CAD build for the part. Positions are in the model's coordinates, mm. Face numbers are marked on the shaded views. A direction names the side the tool comes from. Round coordinates to 2 decimals unless told otherwise and drop trailing zeros. Order: outer loops, then holes, each group sorted by start corner. A loop starts at its lowest first (then second) coordinate and runs counter-clockwise, first axis right, second up. Notation, with made-up numbers: (-4, -35) - (2, -35) arc R26 cw to (2, 0) - close; hole circle Ø8 at (54.5, 3.25). An arc over 180 degrees is marked (long way). Write item = value, one per line.
from build123d import *

# Parameters (mm, degrees)
SKETCH1_W                                 = 101.6
SKETCH1_H                                 = 101.6
BASE_EXTRUDE_DEPTH                        = 3.175
SKETCH9_R                                 = 34.925
CENTER_HOLE_DEPTH                         = 29.575
SKETCH2_R                                 = 5.715
SKETCH2_R_2                               = 3.175
LEFT_HINGE_BASE_DEPTH                     = 50.8
LEFT_HINGE_BASE_DEPTH_BACK                = 50.8
SKETCH2_3_R                               = 3.175
LEFT_HINGE_CUT_DEPTH                      = 50.8
LEFT_HINGE_CUT_DEPTH_BACK                 = 50.8
SKETCH3_W                                 = 101.6
SKETCH3_H                                 = 6.35
LEFT_HINGE_EXTENSION_DEPTH                = 3.503095
SKETCH4_R                                 = 5.715
SKETCH4_R_2                               = 3.175
BACK_HINGE_BASE_DEPTH                     = 50.8
BACK_HINGE_BASE_DEPTH_BACK                = 50.8
SKETCH4_3_R                               = 3.175
BACK_HINGE_CUT_DEPTH                      = 50.8
BACK_HINGE_CUT_DEPTH_BACK                 = 50.8
SKETCH7_W                                 = 101.6
SKETCH7_H                                 = 6.35
BACK_HINGE_EXTENSION_DEPTH                = 3.503095
SKETCH8_W                                 = 13.006904881
SKETCH8_H                                 = 12.7
HINGE_CUT_LEFT_DEPTH                      = 32.115
HINGE_CUT_LEFT_LPATTERN_COUNT             = 4
HINGE_CUT_LEFT_LPATTERN_PITCH             = 25.4
HINGE_CUT_BACK_CIRPATTERN_COUNT           = 2
HINGE_CUT_BACK_CIRPATTERN_ANGLE           = 90
HINGE_CUT_BACK_CIRPATTERN_COPY_1_SKETCH_W = 13.006904881
HINGE_CUT_BACK_CIRPATTERN_COPY_1_SKETCH_H = 12.7
HINGE_CUT_BACK_CIRPATTERN_COPY_1_DEPTH    = 32.115
HINGE_CUT_BACK_CIRPATTERN_COPY_2_SKETCH_W = 13.006904881
HINGE_CUT_BACK_CIRPATTERN_COPY_2_SKETCH_H = 12.7
HINGE_CUT_BACK_CIRPATTERN_COPY_2_DEPTH    = 32.115
HINGE_CUT_BACK_CIRPATTERN_COPY_3_SKETCH_W = 13.006904881
HINGE_CUT_BACK_CIRPATTERN_COPY_3_SKETCH_H = 12.7
HINGE_CUT_BACK_CIRPATTERN_COPY_3_DEPTH    = 32.115
CIRPATTERN2_COPY_1_SKETCH_W               = 13.006904881
CIRPATTERN2_COPY_1_SKETCH_H               = 12.7
CIRPATTERN2_COPY_1_DEPTH                  = 32.115
CIRPATTERN2_COPY_2_SKETCH_W               = 13.006904881
CIRPATTERN2_COPY_2_SKETCH_H               = 12.7
CIRPATTERN2_COPY_2_DEPTH                  = 32.115
CIRPATTERN2_COPY_3_SKETCH_W               = 13.006904881
CIRPATTERN2_COPY_3_SKETCH_H               = 12.7
CIRPATTERN2_COPY_3_DEPTH                  = 32.115
CIRPATTERN2_COPY_4_SKETCH_W               = 13.006904881
CIRPATTERN2_COPY_4_SKETCH_H               = 12.7
CIRPATTERN2_COPY_4_DEPTH                  = 32.115


with BuildPart() as part:
    # Sketch1 → Base Extrude (new body, symmetric)
    with BuildSketch(Plane(origin=(0, 0, 0), x_dir=(1, 0, 0), z_dir=(0, 1, 0))):
        Rectangle(SKETCH1_W, SKETCH1_H)
    extrude(amount=BASE_EXTRUDE_DEPTH, both=True)

    # Sketch9 → Center Hole (cut, through all)
    with BuildSketch(Plane(origin=(0, 25.4, 0), x_dir=(-1, 0, 0), z_dir=(0, 1, 0))):
        with Locations(Location((0, 0, 0), (0, 0, 90))):  # turned: the seam where the file's is
            Circle(SKETCH9_R)
    extrude(amount=-CENTER_HOLE_DEPTH, mode=Mode.SUBTRACT)



with BuildPart() as body_2:
    # Sketch2 → Left Hinge Base (new body, two sides)
    with BuildSketch(Plane.XY) as left_hinge_base_sk:
        with Locations((-59.055, 0)):
            Circle(SKETCH2_R)
        with Locations((-59.055, 0)):
            Circle(SKETCH2_R_2, mode=Mode.SUBTRACT)
        with Locations((-59.055, 0)):
            Circle(SKETCH2_R_2)
    extrude(amount=LEFT_HINGE_BASE_DEPTH)
    extrude(left_hinge_base_sk.sketch, amount=-LEFT_HINGE_BASE_DEPTH_BACK)

    # Sketch2_3 → Left Hinge Cut (cut, two sides)
    with BuildSketch(Plane.XY) as left_hinge_cut_sk:
        with Locations((-59.055, 0)):
            Circle(SKETCH2_3_R)
    extrude(amount=LEFT_HINGE_CUT_DEPTH, mode=Mode.SUBTRACT)
    extrude(left_hinge_cut_sk.sketch, amount=-LEFT_HINGE_CUT_DEPTH_BACK, mode=Mode.SUBTRACT)


with BuildPart() as part_1:
    add(part.part)

    add(body_2.part)  # Left Hinge Extension merges body 2
    # Sketch3 → Left Hinge Extension (add)
    with BuildSketch(Plane.ZY.offset(50.8)):
        Rectangle(SKETCH3_W, SKETCH3_H)
    extrude(amount=LEFT_HINGE_EXTENSION_DEPTH)



with BuildPart() as body_2_2:
    # Sketch4 → Back Hinge Base (new body, two sides)
    with BuildSketch(Plane(origin=(0, 0, 0), x_dir=(0, 0, -1), z_dir=(1, 0, 0))) as back_hinge_base_sk:
        with Locations((59.055, 0)):
            Circle(SKETCH4_R)
        with Locations((59.055, 0)):
            Circle(SKETCH4_R_2, mode=Mode.SUBTRACT)
        with Locations((59.055, 0)):
            Circle(SKETCH4_R_2)
    extrude(amount=BACK_HINGE_BASE_DEPTH)
    extrude(back_hinge_base_sk.sketch, amount=-BACK_HINGE_BASE_DEPTH_BACK)

    # Sketch4_3 → Back Hinge Cut (cut, two sides)
    with BuildSketch(Plane(origin=(0, 0, 0), x_dir=(0, 0, -1), z_dir=(1, 0, 0))) as back_hinge_cut_sk:
        with Locations((59.055, 0)):
            Circle(SKETCH4_3_R)
    extrude(amount=BACK_HINGE_CUT_DEPTH, mode=Mode.SUBTRACT)
    extrude(back_hinge_cut_sk.sketch, amount=-BACK_HINGE_CUT_DEPTH_BACK, mode=Mode.SUBTRACT)


with BuildPart() as part_2:
    add(part_1.part)

    add(body_2_2.part)  # Back Hinge Extension merges body 2 2
    # Sketch7 → Back Hinge Extension (add)
    with BuildSketch(Plane(origin=(0, 0, -50.8), x_dir=(-1, 0, 0), z_dir=(0, 0, -1))):
        Rectangle(SKETCH7_W, SKETCH7_H)
    extrude(amount=BACK_HINGE_EXTENSION_DEPTH)

    # Sketch8 → Hinge Cut Left (cut, through all)
    with BuildSketch(Plane(origin=(0, 25.4, 0), x_dir=(-1, 0, 0), z_dir=(0, 1, 0))):
        with Locations((58.26654756, 44.45)):
            Rectangle(SKETCH8_W, SKETCH8_H)
    hinge_cut_left = extrude(amount=-HINGE_CUT_LEFT_DEPTH, mode=Mode.SUBTRACT)

    # Hinge Cut Left LPattern: Hinge Cut Left ×4
    with Locations(*[(0, 0, -i * HINGE_CUT_LEFT_LPATTERN_PITCH) for i in range(1, HINGE_CUT_LEFT_LPATTERN_COUNT)]):
        add(hinge_cut_left, mode=Mode.SUBTRACT)

    # Hinge Cut Back CirPattern: Hinge Cut Left ×2 about axis
    hinge_cut_back_cirpattern_axis = Axis((0, 0, 0), (0, -1, 0))
    for i in range(1, HINGE_CUT_BACK_CIRPATTERN_COUNT):
        add(hinge_cut_left.rotate(hinge_cut_back_cirpattern_axis, i * HINGE_CUT_BACK_CIRPATTERN_ANGLE / (HINGE_CUT_BACK_CIRPATTERN_COUNT - 1)), mode=Mode.SUBTRACT)

    # Hinge Cut Back CirPattern copy 1 sketch → Hinge Cut Back CirPattern copy 1 (cut, through all)
    with BuildSketch(Plane(origin=(25.4, 25.4, 0), x_dir=(0, 0, -1), z_dir=(0, 1, 0))):
        with Locations((58.26654756, 44.45)):
            Rectangle(HINGE_CUT_BACK_CIRPATTERN_COPY_1_SKETCH_W, HINGE_CUT_BACK_CIRPATTERN_COPY_1_SKETCH_H)
    extrude(amount=-HINGE_CUT_BACK_CIRPATTERN_COPY_1_DEPTH, mode=Mode.SUBTRACT)

    # Hinge Cut Back CirPattern copy 2 sketch → Hinge Cut Back CirPattern copy 2 (cut, through all)
    with BuildSketch(Plane(origin=(50.8, 25.4, 0), x_dir=(0, 0, -1), z_dir=(0, 1, 0))):
        with Locations((58.26654756, 44.45)):
            Rectangle(HINGE_CUT_BACK_CIRPATTERN_COPY_2_SKETCH_W, HINGE_CUT_BACK_CIRPATTERN_COPY_2_SKETCH_H)
    extrude(amount=-HINGE_CUT_BACK_CIRPATTERN_COPY_2_DEPTH, mode=Mode.SUBTRACT)

    # Hinge Cut Back CirPattern copy 3 sketch → Hinge Cut Back CirPattern copy 3 (cut, through all)
    with BuildSketch(Plane(origin=(76.2, 25.4, 0), x_dir=(0, 0, -1), z_dir=(0, 1, 0))):
        with Locations((58.26654756, 44.45)):
            Rectangle(HINGE_CUT_BACK_CIRPATTERN_COPY_3_SKETCH_W, HINGE_CUT_BACK_CIRPATTERN_COPY_3_SKETCH_H)
    extrude(amount=-HINGE_CUT_BACK_CIRPATTERN_COPY_3_DEPTH, mode=Mode.SUBTRACT)

    # CirPattern2 copy 1 sketch → CirPattern2 copy 1 (cut, through all)
    with BuildSketch(Plane(origin=(0, 25.4, 25.4), x_dir=(1, 0, 0), z_dir=(0, 1, 0))):
        with Locations((58.26654756, 44.45)):
            Rectangle(CIRPATTERN2_COPY_1_SKETCH_W, CIRPATTERN2_COPY_1_SKETCH_H)
    extrude(amount=-CIRPATTERN2_COPY_1_DEPTH, mode=Mode.SUBTRACT)

    # CirPattern2 copy 2 sketch → CirPattern2 copy 2 (cut, through all)
    with BuildSketch(Plane(origin=(0, 25.4, 50.8), x_dir=(1, 0, 0), z_dir=(0, 1, 0))):
        with Locations((58.26654756, 44.45)):
            Rectangle(CIRPATTERN2_COPY_2_SKETCH_W, CIRPATTERN2_COPY_2_SKETCH_H)
    extrude(amount=-CIRPATTERN2_COPY_2_DEPTH, mode=Mode.SUBTRACT)

    # CirPattern2 copy 3 sketch → CirPattern2 copy 3 (cut, through all)
    with BuildSketch(Plane(origin=(0, 25.4, 76.2), x_dir=(1, 0, 0), z_dir=(0, 1, 0))):
        with Locations((58.26654756, 44.45)):
            Rectangle(CIRPATTERN2_COPY_3_SKETCH_W, CIRPATTERN2_COPY_3_SKETCH_H)
    extrude(amount=-CIRPATTERN2_COPY_3_DEPTH, mode=Mode.SUBTRACT)

    # CirPattern2 copy 4 sketch → CirPattern2 copy 4 (cut, through all)
    with BuildSketch(Plane(origin=(0, 25.4, 0), x_dir=(1, 0, 0), z_dir=(0, 1, 0))):
        with Locations((58.26654756, 44.45)):
            Rectangle(CIRPATTERN2_COPY_4_SKETCH_W, CIRPATTERN2_COPY_4_SKETCH_H)
    extrude(amount=-CIRPATTERN2_COPY_4_DEPTH, mode=Mode.SUBTRACT)


solid = part_2.part
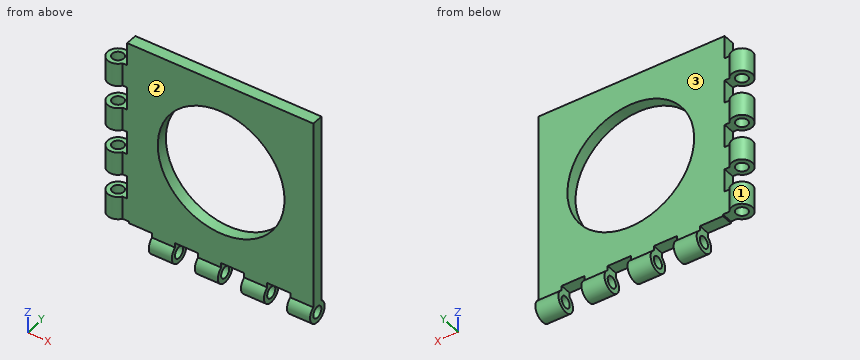
(1) Tool access for the marked faces 1, 2 and 3: list every direction of +Z, -Z, +X, -X, +Y, -Y with a clear straight run to the whole face (end or side of a thin tool).
Solved:
face_1 = +Z, -Z
face_2 = +Z, +X, -Y
face_3 = +Z, +X, +Y
(2) Band-saw the part on B-B on z = -40. List the corners of the cut face in (x, y) (3 decimals), plus the area to 3 significant figures.
Solved:
outline = (-54.303, -3.175) - (50.8, -3.175) - (50.8, 3.175) - (-54.303, 3.175) arc R5.715 ccw (long way) to start; hole circle Ø6.35 at (-59.055, 0)
area = 734 mm²
(3) Band-saw the part on A-A on x = -17. List the corners of the cut face in (y, z) (3 decimals).
Solved:
outline = (-3.175, -51.763) - (3.175, -51.763) - (3.175, -30.508) - (-3.175, -30.508) - close; (-3.175, 30.508) - (3.175, 30.508) - (3.175, 50.8) - (-3.175, 50.8) - close
(4) Probe line 1 along X through (y, z) = (-4.25, -57.5); line 2 along Z through (x, y) = (-2, 2); line 3 along X through (y, z) = (0, 3). List the from-to ranges inside material, lowest first.
Solved:
line_1 = -38.1 to -25.4, -12.7 to 0, 12.7 to 25.4, 38.1 to 50.8
line_2 = -64.41 to -61.52, -56.59 to -34.87, 34.87 to 50.8
line_3 = -64.77 to -62.23, -55.88 to -34.8, 34.8 to 50.8
(5) Drop flat-ended pins along their axis: pin 1 (1.9 mm diameter, centred on x = 33, y = -0.5, fed in from -Z); pin 2 (5 mm diameter, centred on y = -0.5, z = 14.5, fed in from -X); pin 3 (5 mm diameter, centred on y = -1, z = -6.5, fed in from -X); pin 4 (4 mm diameter, centred on x = -32.5, z = 35, fed in from +Y) (3 decimals). Give the stop position or say it passes through.
Solved:
pin_1 = -51.76
pin_2 = -64.77
pin_3 = -51.76
pin_4 = 3.175
